Check sheet for the modelled part. Datum: model origin and axes. Units: mm. Coordinates: 2 decimals unless noted, no trailing zeros. Write each loop counter-clockwise with the first axis right and the second up, starting at its lowest first coordinate (ties: lowest second). Pieces come first, ordered by that corner, then holes. Notation, with made-up numbers: (52.25, 84.25) -> (63.25, 84.25) arc R28 cw to (63.25, 122.25) -> close; hole circle Ø1 at (43, 1.25). An arc over 180 degrees is marked (long way). Put each result on its own line as item: value.
```python
from build123d import *

# Parameters (mm, degrees)
SKETCH1_R           = 1.625
SKETCH1_W           = 20
SKETCH1_H           = 10
BOSS_EXTRUDE1_DEPTH = 4
FILLET1_R           = 2


with BuildPart() as part:
    # Sketch1 → Boss-Extrude1 (new body)
    with BuildSketch(Plane.XY):
        Polygon((-35.731071717, 115.203558257), (4, 81.865230633), (4, -4), (-120, -4), (-120, 0), (-120, 20.998655539), (-38.79524949, 117.774708696), align=None)
        with Locations((-5, 5)):
            Circle(SKETCH1_R, mode=Mode.SUBTRACT)
        with Locations((-111, 5)):
            Circle(SKETCH1_R, mode=Mode.SUBTRACT)
        with Locations((-111, 17)):
            Circle(SKETCH1_R, mode=Mode.SUBTRACT)
        with Locations((-37.685937989, 105.09522022)):
            Circle(SKETCH1_R, mode=Mode.SUBTRACT)
        with Locations((-5, 77.668461709)):
            Circle(SKETCH1_R, mode=Mode.SUBTRACT)
        with Locations((-91, 5)):
            Rectangle(SKETCH1_W, SKETCH1_H, mode=Mode.SUBTRACT)
    extrude(amount=BOSS_EXTRUDE1_DEPTH)

    # Fillet1
    fillet1_edges = [part.edges().sort_by_distance(p)[0] for p in [
        (-101, 10, 2),
        (-101, 0, 2),
        (-81, 0, 2),
        (-81, 10, 2),
    ]]
    fillet(fillet1_edges, radius=FILLET1_R)


solid = part.part
```
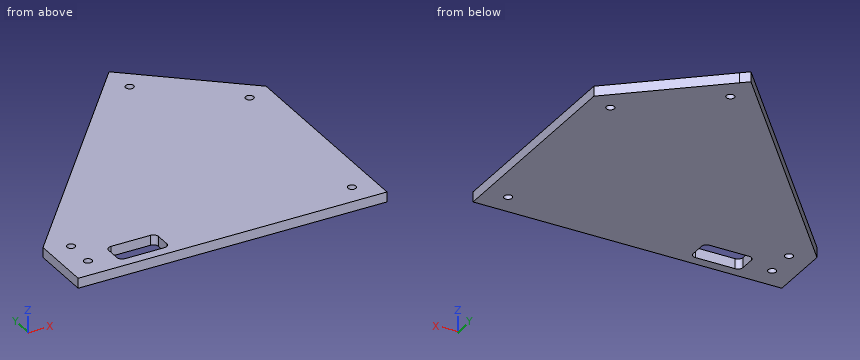
Q1. Cross-section at D-D (x = -5). Record the cut outline in (y, z) (3 decimals), plus the area to 3 significant figures.
Recorded:
outline: (-4, 0) -> (3.375, 0) -> (3.375, 4) -> (-4, 4) -> close; (6.625, 0) -> (76.043, 0) -> (76.043, 4) -> (6.625, 4) -> close; (79.293, 0) -> (89.417, 0) -> (89.417, 4) -> (79.293, 4) -> close
area: 348 mm2
Q2. Material ranges on line 1 along Y through (x, z) = (-111, 2.6) (3 decimals); line 2 along Y through (x, z) = (-5, 2.9) (3 decimals); line 3 along Y through (x, z) = (-84.5, 2), recorded low to high.
Recorded:
line 1: y = -4 to 3.375, 6.625 to 15.375, 18.625 to 31.724
line 2: y = -4 to 3.375, 6.625 to 76.043, 79.293 to 89.417
line 3: y = -4 to 0, 10 to 63.31
Q3. Depth check by flat-ended pin: P1, Ø4, axis at x = -52.5, y = 45, coming from the -Z side. Enter the tip coordinate at first touch or a pass-through.
Recorded:
P1: stops at z = 0
Q4. Cross-section at A-A (y = 5). Record the cut outline in (x, z) (3 decimals), plus the area to 3 significant figures.
Recorded:
outline: (-120, 0) -> (-112.625, 0) -> (-112.625, 4) -> (-120, 4) -> close; (-109.375, 0) -> (-101, 0) -> (-101, 4) -> (-109.375, 4) -> close; (-81, 0) -> (-6.625, 0) -> (-6.625, 4) -> (-81, 4) -> close; (-3.375, 0) -> (4, 0) -> (4, 4) -> (-3.375, 4) -> close
area: 390 mm2
Q5. Cross-section at B-B (x = -111). Record the cut outline in (y, z) (3 decimals), plus the area to 3 significant figures.
Recorded:
outline: (-4, 0) -> (3.375, 0) -> (3.375, 4) -> (-4, 4) -> close; (6.625, 0) -> (15.375, 0) -> (15.375, 4) -> (6.625, 4) -> close; (18.625, 0) -> (31.724, 0) -> (31.724, 4) -> (18.625, 4) -> close
area: 117 mm2
Q6. Cross-section at C-C (z = 2.2). Record the cut outline in (x, y) (3 decimals).
Recorded:
outline: (-120, -4) -> (4, -4) -> (4, 81.865) -> (-38.795, 117.775) -> (-120, 20.999) -> close; hole circle Ø3.25 at (-111, 5); hole circle Ø3.25 at (-111, 17); hole (-101, 2) arc R2 ccw to (-99, 0) -> (-83, 0) arc R2 ccw to (-81, 2) -> (-81, 8) arc R2 ccw to (-83, 10) -> (-99, 10) arc R2 ccw to (-101, 8) -> close; hole circle Ø3.25 at (-37.686, 105.095); hole circle Ø3.25 at (-5, 5); hole circle Ø3.25 at (-5, 77.668)
